Verification items for the finished model (mm, model axes). Face numbers are marked on the shaded views. Coordinates: 2 decimals unless noted, no trailing zeros. Loops run counter-clockwise (first coordinate to the right, second up) from the corner with the lowest first, then second, coordinate; pieces in that order, holes last. Notation, with made-up numbers: (9.5, 72) - (47.5, 72) arc R14 ccw to (47.5, 98) - close; hole circle Ø8 at (6, 23). An arc over 180 degrees is marked (long way). One line per item, written item: value. Start each with the question number.
(1) Section check B-B (x = -106). Record the boundary of the cut face in (y, z).
(2) Gauge pin test, flat end, axial feed: P1, Ø1, axis at x = 66, y = -1, coming from the -Z side. Record the tip position at first contact, or that the pin passes through.
(3) Draft check along X on the marked faces 1 and 2. Enter one of: +X half, -X half, draft (parallel to the pull), parting line (faces both ways), or undercut.
(4) Section check A-A (z = 38). Record the boundary of the cut face in (x, y), plus the area to 4 significant figures.
(5) Thickness scan on probe 1 along X at (y, z) = (-2.25, 98.5); probe 2 along X at (y, z) = (-0.25, 71); probe 3 along X at (y, z) = (-5, 59). Record the ranges inside material, lowest first. Write a range as [from, to].
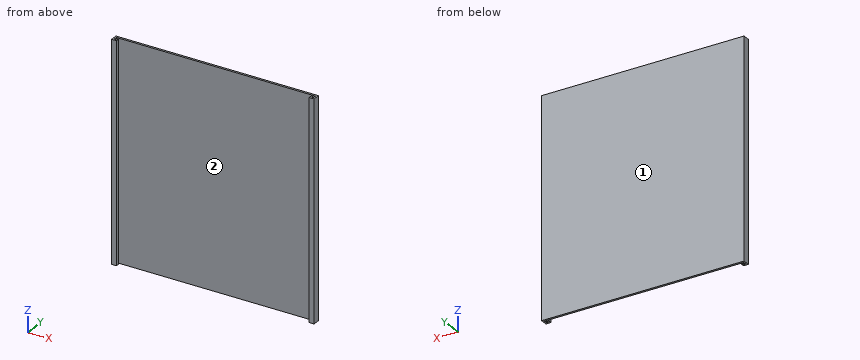
```python
from build123d import *

# Parameters (mm, degrees)
SKETCH2_W                = 243
SKETCH2_H                = 265
BOSS_EXTRUDE1_DEPTH      = 2.5
BOSS_EXTRUDE2_DEPTH      = 4
BOSS_EXTRUDE2_DEPTH_BACK = 2.5
SKETCH3_W                = 2
SKETCH3_H                = 265
BOSS_EXTRUDE3_DEPTH      = 4
BOSS_EXTRUDE3_DEPTH_BACK = 2.5
SKETCH4_W                = 2
SKETCH4_H                = 265
BOSS_EXTRUDE4_DEPTH      = 2
BOSS_EXTRUDE4_DEPTH_BACK = 2
SKETCH5_W                = 265
SKETCH5_H                = 2
BOSS_EXTRUDE5_DEPTH      = 2
BOSS_EXTRUDE5_DEPTH_BACK = 2
SKETCH6_W                = 265
SKETCH6_H                = 2
SKETCH7_W                = 2
SKETCH7_H                = 265
BOSS_EXTRUDE7_DEPTH      = 4
SKETCH8_W                = 2
SKETCH8_H                = 265
BOSS_EXTRUDE8_DEPTH      = 4


with BuildPart() as part:
    # Sketch2 → Boss-Extrude1 (new body)
    with BuildSketch(Plane(origin=(0, 0, 0), x_dir=(1, 0, 0), z_dir=(0, 1, 0))):
        Rectangle(SKETCH2_W, SKETCH2_H)
    extrude(amount=BOSS_EXTRUDE1_DEPTH)

    # Sketch3 → Boss-Extrude2 (add, two sides: drawn at the far end of the back side and taken through both)
    with BuildSketch(Plane.XZ.offset(-BOSS_EXTRUDE2_DEPTH_BACK)):
        with Locations((122.5, 0)):
            Rectangle(SKETCH3_W, SKETCH3_H)
    extrude(amount=BOSS_EXTRUDE2_DEPTH + BOSS_EXTRUDE2_DEPTH_BACK)

    # Sketch4 → Boss-Extrude3 (add, two sides: drawn at the far end of the back side and taken through both)
    with BuildSketch(Plane.XZ.offset(-BOSS_EXTRUDE3_DEPTH_BACK)):
        with Locations((-122.5, 0)):
            Rectangle(SKETCH4_W, SKETCH4_H)
    extrude(amount=BOSS_EXTRUDE3_DEPTH + BOSS_EXTRUDE3_DEPTH_BACK)

    # Sketch5 → Boss-Extrude4 (add, two sides: drawn at the far end of the back side and taken through both)
    with BuildSketch(Plane(origin=(-121.5, 0, 0), x_dir=(0, 0, -1), z_dir=(1, 0, 0)).offset(-BOSS_EXTRUDE4_DEPTH_BACK)):
        with Locations((0, -5)):
            Rectangle(SKETCH5_W, SKETCH5_H)
    extrude(amount=BOSS_EXTRUDE4_DEPTH + BOSS_EXTRUDE4_DEPTH_BACK)

    # Sketch6 → Boss-Extrude5 (add, two sides: drawn at the far end of the back side and taken through both)
    with BuildSketch(Plane.ZY.offset(-121.5).offset(-BOSS_EXTRUDE5_DEPTH_BACK)):
        with Locations((0, -5)):
            Rectangle(SKETCH6_W, SKETCH6_H)
    extrude(amount=BOSS_EXTRUDE5_DEPTH + BOSS_EXTRUDE5_DEPTH_BACK)

    # Sketch7 → Boss-Extrude7 (add)
    with BuildSketch(Plane.XZ.offset(6)):
        with Locations((118.5, 0)):
            Rectangle(SKETCH7_W, SKETCH7_H)
    extrude(amount=-BOSS_EXTRUDE7_DEPTH)

    # Sketch8 → Boss-Extrude8 (add)
    with BuildSketch(Plane.XZ.offset(6)):
        with Locations((-118.5, 0)):
            Rectangle(SKETCH8_W, SKETCH8_H)
    extrude(amount=-BOSS_EXTRUDE8_DEPTH)


solid = part.part
```
Responses:
1. outline: (0, -132.5) - (2.5, -132.5) - (2.5, 132.5) - (0, 132.5) - close
2. P1: passes through
3. face 1: draft
3. face 2: undercut
4. outline: (-123.5, -6) - (-117.5, -6) - (-117.5, -2) - (-119.5, -2) - (-119.5, -4) - (-121.5, -4) - (-121.5, 0) - (121.5, 0) - (121.5, -4) - (119.5, -4) - (119.5, -2) - (117.5, -2) - (117.5, -6) - (123.5, -6) - (123.5, 2.5) - (-123.5, 2.5) - close
4. area: 665.5 mm²
5. probe 1: x = [-123.5, -121.5], [-119.5, -117.5], [117.5, 119.5], [121.5, 123.5]
5. probe 2: x = [-123.5, -121.5], [121.5, 123.5]
5. probe 3: x = [-123.5, -117.5], [117.5, 123.5]
